CAD build for the part. Positions are in the model's coordinates, mm. Face numbers are marked on the shaded views. A direction names the side the tool comes from. Round coordinates to 2 decimals unless told otherwise and drop trailing zeros. Loops run counter-clockwise (first coordinate to the right, second up) from the corner with the lowest first, then second, coordinate; pieces in that order, holes last.
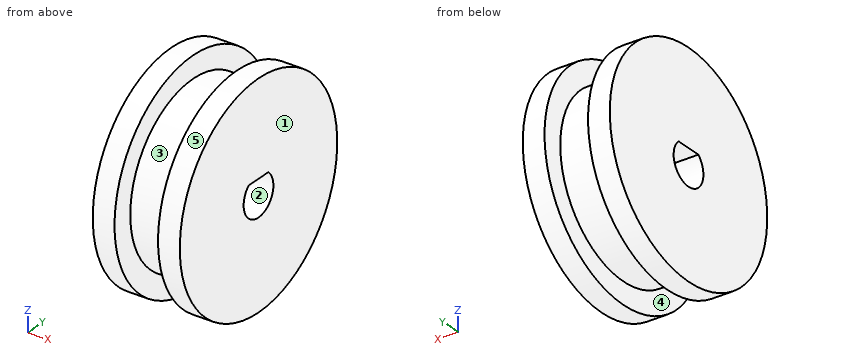
from build123d import *

# Parameters (mm, degrees)
F3_DEPTH      = 6.35
F3_DEPTH_BACK = 6.35


with BuildPart() as f1:
    # F0 (on Front) → F1 (revolve)
    with BuildSketch(Plane.XZ):
        Polygon((-6.35, 15.875), (-6.35, 3), (6.35, 3), (6.35, 15.875), (3.175, 15.875), (3.175, 12.7), (-3.175, 12.7), (-3.175, 15.875), align=None)
    revolve(axis=Axis((0, 0, 0), (1, 0, 0)))

    # F2 (on Right) → F3 (join, two sides)
    with BuildSketch(Plane.YZ) as f3_sk:
        with BuildLine():
            Line((-1.9843134833, 2.25), (1.9843134833, 2.25))
            ThreePointArc((1.9843134833, 2.25), (0, 3), (-1.9843134833, 2.25))
        make_face()
    extrude(amount=F3_DEPTH)
    extrude(f3_sk.sketch, amount=-F3_DEPTH_BACK)


solid = f1.part
Item 1: Cut at A-A (z = 0). List the corners of the cut face in (x, y) (3 decimals), plus the area to 3 significant figures.
Verdict:
outline: (-6.35, -15.875) - (-3.175, -15.875) - (-3.175, -12.7) - (3.175, -12.7) - (3.175, -15.875) - (6.35, -15.875) - (6.35, -3) - (-6.35, -3) - close; (-6.35, 3) - (6.35, 3) - (6.35, 15.875) - (3.175, 15.875) - (3.175, 12.7) - (-3.175, 12.7) - (-3.175, 15.875) - (-6.35, 15.875) - close
area: 287 mm2
Item 2: Mould opens along Z. For the marked faces 1, 2 and 3 say: released by +Z, released by -Z, zero draft, split by the parting line, or undercut.
Verdict:
face 1: zero draft
face 2: undercut
face 3: split by the parting line
Item 3: Cut at B-B (y = 0). List the corners of the cut face in (x, z) (3 decimals), plus the area to 3 significant figures.
Verdict:
outline: (-6.35, -15.875) - (-3.175, -15.875) - (-3.175, -12.7) - (3.175, -12.7) - (3.175, -15.875) - (6.35, -15.875) - (6.35, -3) - (-6.35, -3) - close; (-6.35, 2.25) - (6.35, 2.25) - (6.35, 15.875) - (3.175, 15.875) - (3.175, 12.7) - (-3.175, 12.7) - (-3.175, 15.875) - (-6.35, 15.875) - close
area: 296 mm2
Item 4: 3-axis set-ups, long thin cutter, end or side, ignore diameter. For the marked faces 4 and 5: which of +Z, -Z, +X, -X, +Y, -Y reach the whole face in a straight line?
Verdict:
face 4: none
face 5: +X, -X
Item 5: Cut at D-D (z = 9). List the corners of the cut face in (x, y) (3 decimals), plus the area to 3 significant figures.
Verdict:
outline: (-6.35, -13.077) - (-3.175, -13.077) - (-3.175, -8.96) - (3.175, -8.96) - (3.175, -13.077) - (6.35, -13.077) - (6.35, 13.077) - (3.175, 13.077) - (3.175, 8.96) - (-3.175, 8.96) - (-3.175, 13.077) - (-6.35, 13.077) - close
area: 280 mm2
Item 6: Flat gauge pins, fed straight in: P1, Ø5, axis at x = 4.5, y = -9, coming from the +Z side; P2, Ø2, axis at x = -3.5, z = -2.5, coming from the +Y side; P3, Ø1.5, axis at x = 0.5, y = 2.5, coming from the +Z side. Where does each tip first touch, or does it go through?
Verdict:
P1: stops at z = 14.48
P2: stops at y = 15.8
P3: stops at z = 12.58
Item 7: Cut at C-C (x = 1.5). List the corners of the cut face in (y, z).
Verdict:
outline: circle Ø25.4 at (0, 0); hole (-1.98, 2.25) arc R3 ccw (long way) to (1.98, 2.25) - close
Item 8: Wall check: L1, parallel to Y at x = -1.5, z = 0; L2, parallel to Y at x = -3.5, z = 0 (3 decimals); L3, parallel to X at y = -8.5, z = -11 (3 decimals). Give the ranges that are in metal, low to high.
Verdict:
L1: y = -12.7 to -3, 3 to 12.7
L2: y = -15.875 to -3, 3 to 15.875
L3: x = -6.35 to -3.175, 3.175 to 6.35
